from build123d import *

# Parameters (mm, degrees)
F0_R     = 2.54
F1_DEPTH = 3.175


# Not quite as in the source:
# - a length typed as a fraction of an inch, garbled in the dataset ("3 / 203.2 mm" for 3/8 in), is restored


with BuildPart() as f1:
    # F0 (on Top) → F1 (new body)
    with BuildSketch(Plane.XY):
        Polygon((139.7, 101.6), (0, 101.6), (0, 25.4), (25.4, 25.4), (25.4, 0), (114.3, 0), (114.3, 25.4), (139.7, 25.4), align=None)
        with Locations((91.775, 77.55)):
            Circle(F0_R, mode=Mode.SUBTRACT)
        with Locations((91.775, 87.55)):
            Circle(F0_R, mode=Mode.SUBTRACT)
        Polygon((94.775, 92.55), (104.775, 92.55), (129.775, 92.55), (129.775, 72.55), (104.775, 72.55), (94.775, 72.55), align=None, mode=Mode.SUBTRACT)
        with Locations((132.775, 77.55)):
            Circle(F0_R, mode=Mode.SUBTRACT)
        with Locations((132.775, 87.55)):
            Circle(F0_R, mode=Mode.SUBTRACT)
    extrude(amount=F1_DEPTH)


solid = f1.part
The listing builds one solid part. Answer for the finished solid, in the listing's coordinates (mm). A direction names the side the tool comes from. Round coordinates to 2 decimals unless told otherwise and drop trailing zeros. Loops run counter-clockwise (first coordinate to the right, second up) from the corner with the lowest first, then second, coordinate; pieces in that order, holes last. Notation, with made-up numbers: M -0.5,72.5 L 54.5,72.5 A20 cw 54.5,92.5 Z; hole C 64,15 d2. An arc over 180 degrees is marked long. Return JSON: item names as keys, results as strings.
Q1. Find section B-B, the plane y = 87.55. Determine the outline of the cut face in (x, z) (3 decimals).
Results list:
{"outline": "M 0,0 L 89.235,0 L 89.235,3.175 L 0,3.175 Z; M 94.315,0 L 94.775,0 L 94.775,3.175 L 94.315,3.175 Z; M 129.775,0 L 130.235,0 L 130.235,3.175 L 129.775,3.175 Z; M 135.315,0 L 139.7,0 L 139.7,3.175 L 135.315,3.175 Z"}
Q2. Each of these flat-tipped pins is pushed along its axis until it touches: pin 1 Ø1.6 at (x, z) = (121, 2.5) entering from -Y; pin 2 Ø1 at (y, z) = (18, 1.5) entering from +X. Where does it stop, or does it pass through?
Results list:
{"pin 1": "stops at y = 25.4", "pin 2": "stops at x = 114.3"}
Q3. Find the intervals of material crossed by line 1 along Y through (x, z) = (129, 0.35); line 2 along X through (y, z) = (79.5, 2.8) (3 decimals); line 3 along Y through (x, z) = (102.5, 1.45), in increasing order. Write a range as from..to.
Results list:
{"line 1": "y = 25.4..72.55, 92.55..101.6", "line 2": "x = 0..90.147, 93.403..94.775, 129.775..131.147, 134.403..139.7", "line 3": "y = 0..72.55, 92.55..101.6"}
Q4. Which of the six approach directions +Z, -Z, +X, -X, +Y, -Y give full straight-line access (tool end or side, diameter ignored) to faces 1 (the face through (69, 52, 3.175)), 2 (the face through (13, 25.4, 2)), 3 (the face through (112, 92.55, 2))?
Results list:
{"face 1": "+Z, +X, -X, +Y, -Y", "face 2": "+Z, -Z, -X, -Y", "face 3": "+Z, -Z"}
Q5. Find section C-C, the plane z = 2.35. Determine the outline of the cut face in (x, y) (3 decimals), plus the area to 3 significant figures.
Results list:
{"outline": "M 0,25.4 L 25.4,25.4 L 25.4,0 L 114.3,0 L 114.3,25.4 L 139.7,25.4 L 139.7,101.6 L 0,101.6 Z; hole C 91.775,77.55 d5.08; hole C 91.775,87.55 d5.08; hole M 94.775,72.55 L 129.775,72.55 L 129.775,92.55 L 94.775,92.55 Z; hole C 132.775,77.55 d5.08; hole C 132.775,87.55 d5.08", "area": "12,100 mm2"}
Q6. Find section A-A, the plane x = 98. Determine the outline of the cut face in (y, z) (3 decimals).
Results list:
{"outline": "M 0,0 L 72.55,0 L 72.55,3.175 L 0,3.175 Z; M 92.55,0 L 101.6,0 L 101.6,3.175 L 92.55,3.175 Z"}
Q7. The mould has two halves that part along X. Classify faces 4 (the face through (127, 25.4, 2)), 5 (the face through (25.4, 13, 2)), 6 (the face through (134.14, 89.69, 1.57)), 7 (the face through (114.3, 13, 2)): released by +X, released by -X, zero draft, split by the parting line, or undercut.
Results list:
{"face 4": "zero draft", "face 5": "released by -X", "face 6": "undercut", "face 7": "released by +X"}
Q8. Find section D-D, the plane y = 10.5. Determine the outline of the cut face in (x, z) (3 decimals), plus the area to 3 significant figures.
Results list:
{"outline": "M 25.4,0 L 114.3,0 L 114.3,3.175 L 25.4,3.175 Z", "area": "282 mm2"}
